Geometry check sheet. Reference: the model listing, model coordinates, mm. A direction names the side the tool comes from. Coordinates: 2 decimals unless noted, no trailing zeros. Write each loop counter-clockwise with the first axis right and the second up, starting at its lowest first coordinate (ties: lowest second). Pieces come first, ordered by that corner, then holes. Notation, with made-up numbers: (60, 37) -> (98, 37) arc R7 ccw to (98, 48) -> close; hole circle Ø10 at (37, 16.5). An arc over 180 degrees is marked (long way). Put each result on its own line as item: value. Start each with the question number.
from build123d import *

# Parameters (mm, degrees)
F1_W      = 4
F1_H      = 4
F2_DEPTH  = 2.5
F3_R      = 2
F4_DEPTH  = 15
F5_R      = 2
F6_DEPTH  = 15
F7_R      = 2
F8_DEPTH  = 15
F9_R      = 1.5
F10_DEPTH = 35.001
F11_R     = 1.5
F12_DEPTH = 16


with BuildPart() as f2:
    # F1 (on Top) → F2 (new body, symmetric)
    with BuildSketch(Plane.XY):
        Rectangle(F1_W, F1_H)
    extrude(amount=F2_DEPTH, both=True)

    # F3 (on face) → F4 (join)
    with BuildSketch(Plane.XY.offset(2.5)):
        Circle(F3_R)
    extrude(amount=F4_DEPTH)

    # F5 (on face) → F6 (join)
    with BuildSketch(Plane(origin=(0, 0, -2.5), x_dir=(1, 0, 0), z_dir=(0, 0, -1))):
        Circle(F5_R)
    extrude(amount=F6_DEPTH)

    # F7 (on face) → F8 (join)
    with BuildSketch(Plane.YZ.offset(2)):
        Circle(F7_R)
    extrude(amount=F8_DEPTH)

    # F9 (on face) → F10 (cut, through all)
    with BuildSketch(Plane.XY.offset(17.5)):
        Circle(F9_R)
    extrude(amount=-F10_DEPTH, mode=Mode.SUBTRACT)

    # F11 (on face) → F12 (cut)
    with BuildSketch(Plane.YZ.offset(17)):
        Circle(F11_R)
    extrude(amount=-F12_DEPTH, mode=Mode.SUBTRACT)


solid = f2.part
Item 1: Go/stop test with flat-tipped pins: P1, Ø1.8, axis at x = 0, y = 0, coming from the -Z side; P2, Ø2, axis at y = -0.5, z = -8, coming from the +X side; P3, Ø2, axis at x = 5, y = 0.5, coming from the -Z side. Record where each tip stops, or that it passes through.
Item 2: Scan lines: line 1 along Z through (x, y) = (13.25, 0); line 2 along Y through (x, z) = (1.25, 13). Record each from-to range of solid material in increasing order. Write a range as [from, to].
Item 3: Section check A-A, the plane z = 9.5. Enter the section's corners in (x, y), and give its area (3 significant figures).
Item 4: Mould release check, pull along X, two halves, no side actions. Record for faces 1 (the flat face through (1.6, -1.6, 2.5)), 2 (the cylindrical face through (-1.5, 0.07, 0.25)), 3 (the flat face through (2, -0.5, 2.1)): released by +X, released by -X, zero draft, split by the parting line, or undercut.
Item 5: Section check B-B, the plane y = 0.45. Enter the section's corners in (x, z), and give its area (3 significant figures).
Item 6: Access from +Z, -Z, +X, -X, +Y, -Y to the whole of each face (thin tool, end or side, straight path). Record for faces 4 (the flat face through (1.5, 1.6, -2.5)), 5 (the cylindrical face through (9, 0, -2)), 6 (the flat face through (-1.6, -1.5, 2.5)), 7 (the cylindrical face through (0, -2, 10)).
From the geometry:
1. P1: through
1. P2: x = 2
1. P3: z = -2
2. line 1: [-2, -1.5], [1.5, 2]
2. line 2: [-1.56, -0.83], [0.83, 1.56]
3. outline: circle Ø4 at (0, 0); hole circle Ø3 at (0, 0)
3. area: 5.50 mm²
4. face 1: zero draft
4. face 2: undercut
4. face 3: released by +X
5. outline: (-2, -2.5) -> (-1.95, -2.5) -> (-1.95, -17.5) -> (-1.43, -17.5) -> (-1.43, 17.5) -> (-1.95, 17.5) -> (-1.95, 2.5) -> (-2, 2.5) -> close; (1.43, -17.5) -> (1.95, -17.5) -> (1.95, -2.5) -> (2, -2.5) -> (2, -1.95) -> (17, -1.95) -> (17, -1.43) -> (1.43, -1.43) -> close; (1.43, 1.43) -> (17, 1.43) -> (17, 1.95) -> (2, 1.95) -> (2, 2.5) -> (1.95, 2.5) -> (1.95, 17.5) -> (1.43, 17.5) -> close
5. area: 50.7 mm²
6. face 4: -Z, +X, +Y
6. face 5: +X
6. face 6: +Z, -X, -Y
6. face 7: +Z
